```python
from build123d import *

# Parameters (mm, degrees)
SKETCH1_R             = 90
BOSS_EXTRUDE1_DEPTH   = 30
CUT_EXTRUDE4_DEPTH    = 30
SKETCH5_R             = 55.626023842
CUT_EXTRUDE5_DEPTH    = 30
SKETCH6_W             = 7.386739777
SKETCH6_H             = 13.542356258
CUT_EXTRUDE6_DEPTH    = 30
FILLET1_R             = 10
SKETCH8_R             = 10.49811893
BOSS_EXTRUDE2_DEPTH   = 30
BOSS_EXTRUDE2_2_DEPTH = 30
BOSS_EXTRUDE2_3_DEPTH = 30
BOSS_EXTRUDE2_4_DEPTH = 30
BOSS_EXTRUDE2_5_DEPTH = 30
BOSS_EXTRUDE4_DEPTH   = 30


with BuildPart() as part:
    # Sketch1 → Boss-Extrude1 (new body)
    with BuildSketch(Plane.XY):
        Circle(SKETCH1_R)
    extrude(amount=BOSS_EXTRUDE1_DEPTH)

    # Sketch4 → Cut-Extrude4 (cut)
    with BuildSketch(Plane.XY):
        with BuildLine():
            Line((88.736574157, 15.027322012), (45.122701232, 44.870398789))
            Line((45.122701232, 44.870398789), (52.120312028, 73.372154623))
            ThreePointArc((52.120312028, 73.372154623), (76.231197482, 47.84145201), (88.736574157, 15.027322012))
        make_face()
        with BuildLine():
            Line((41.712941959, -79.749799204), (56.61796667, -29.048523269))
            Line((56.61796667, -29.048523269), (85.887127938, -26.896119693))
            ThreePointArc((85.887127938, -26.896119693), (69.056660207, -57.716355404), (41.712941959, -79.749799204))
        make_face()
        with BuildLine():
            Line((-62.956558256, -64.315408516), (-10.130873456, -62.823373493))
            Line((-10.130873456, -62.823373493), (0.960852233, -89.994870759))
            ThreePointArc((0.960852233, -89.994870759), (-33.551834325, -83.512121356), (-62.956558256, -64.315408516))
        make_face()
        with BuildLine():
            Line((-80.622234776, 40.000690741), (-62.879190802, -9.778456837))
            Line((-62.879190802, -9.778456837), (-85.2932886, -28.723769249))
            ThreePointArc((-85.2932886, -28.723769249), (-89.792834204, 6.103025933), (-80.622234776, 40.000690741))
        make_face()
        with BuildLine():
            Line((13.129276916, 89.037194967), (-28.730603645, 56.77995481))
            Line((-28.730603645, 56.77995481), (-53.6750036, 72.242605078))
            ThreePointArc((-53.6750036, 72.242605078), (-21.943189159, 87.283998817), (13.129276916, 89.037194967))
        make_face()
    extrude(amount=CUT_EXTRUDE4_DEPTH, mode=Mode.SUBTRACT)

    # Sketch5 → Cut-Extrude5 (cut)
    with BuildSketch(Plane.XY):
        Circle(SKETCH5_R)
    extrude(amount=CUT_EXTRUDE5_DEPTH, mode=Mode.SUBTRACT)

    # Sketch6 → Cut-Extrude6 (cut)
    with BuildSketch(Plane.XY):
        with Locations((56.030331415, 2.229633356)):
            Rectangle(SKETCH6_W, SKETCH6_H)
    extrude(amount=CUT_EXTRUDE6_DEPTH, mode=Mode.SUBTRACT)

    # Fillet1
    fillet1_edges = [part.edges().sort_by_distance(p)[0] for p in [
        (85.887127938, -26.896119693, 15),
        (0.960852233, -89.994870759, 15),
        (-85.2932886, -28.723769249, 15),
        (-53.6750036, 72.242605078, 15),
        (52.120312028, 73.372154623, 15),
    ]]
    fillet(fillet1_edges, radius=FILLET1_R)



with BuildPart() as body_2:
    # Sketch8 → Boss-Extrude2 (new body)
    with BuildSketch(Plane.XY.offset(30)):
        with Locations((67.093562258, 42.627771692)):
            Circle(SKETCH8_R)
    extrude(amount=-BOSS_EXTRUDE2_DEPTH)


with BuildPart() as body_3:
    # Sketch8 → Boss-Extrude2 2 (new body)
    with BuildSketch(Plane.XY.offset(30)):
        with Locations((61.274470993, -50.637063702)):
            Circle(SKETCH8_R)
    extrude(amount=-BOSS_EXTRUDE2_2_DEPTH)


with BuildPart() as body_4:
    # Sketch8 → Boss-Extrude2 3 (new body)
    with BuildSketch(Plane.XY.offset(30)):
        with Locations((-29.223856541, -73.92319815)):
            Circle(SKETCH8_R)
    extrude(amount=-BOSS_EXTRUDE2_3_DEPTH)


with BuildPart() as body_5:
    # Sketch8 → Boss-Extrude2 4 (new body)
    with BuildSketch(Plane.XY.offset(30)):
        with Locations((-79.335807618, 4.950014688)):
            Circle(SKETCH8_R)
    extrude(amount=-BOSS_EXTRUDE2_4_DEPTH)


with BuildPart() as body_6:
    # Sketch8 → Boss-Extrude2 5 (new body)
    with BuildSketch(Plane.XY.offset(30)):
        with Locations((-19.808369092, 76.982475472)):
            Circle(SKETCH8_R)
    extrude(amount=-BOSS_EXTRUDE2_5_DEPTH)


with BuildPart() as part_1:
    add(part.part)

    add(body_2.part)  # Boss-Extrude4 merges body 2

    add(body_3.part)  # Boss-Extrude4 merges body 3

    add(body_4.part)  # Boss-Extrude4 merges body 4

    add(body_5.part)  # Boss-Extrude4 merges body 5

    add(body_6.part)  # Boss-Extrude4 merges body 6
    # Sketch9 → Boss-Extrude4 (add)
    with BuildSketch(Plane.XY):
        with BuildLine():
            Line((-29.298411126, 72.493644527), (-38.186452488, 62.641490221))
            Line((-38.186452488, 62.641490221), (-33.742460025, 59.886727574))
            Line((-33.742460025, 59.886727574), (-26.440954647, 68.84495067))
            ThreePointArc((-26.440954647, 68.84495067), (-28.073538286, 70.509649254), (-29.298411126, 72.493644527))
        make_face()
        with BuildLine():
            Line((46.528668919, 50.597003041), (57.304734615, 46.421101948))
            ThreePointArc((57.304734615, 46.421101948), (58.383460962, 48.48820141), (59.891846071, 50.266212961))
            Line((59.891846071, 50.266212961), (47.775334692, 55.674759504))
            Line((47.775334692, 55.674759504), (46.528668919, 50.597003041))
        make_face()
        with BuildLine():
            Line((62.498758869, -28.616059966), (61.857228356, -40.15513187))
            ThreePointArc((61.857228356, -40.15513187), (64.156501542, -40.54229273), (66.313607647, -41.427416431))
            Line((66.313607647, -41.427416431), (67.713233152, -28.232596532))
            Line((67.713233152, -28.232596532), (62.498758869, -28.616059966))
        make_face()
        with BuildLine():
            Line((-7.902311684, -68.282700724), (-19.074865041, -71.238338267))
            ThreePointArc((-19.074865041, -71.238338267), (-18.73256241, -73.544716298), (-18.907782629, -75.869764382))
            Line((-18.907782629, -75.869764382), (-5.926255116, -73.123463752))
            Line((-5.926255116, -73.123463752), (-7.902311684, -68.282700724))
        make_face()
        with BuildLine():
            Line((-67.382656079, -13.584969925), (-73.646143282, -3.872582481))
            ThreePointArc((-73.646143282, -3.872582481), (-75.733861807, -4.910841636), (-77.999259963, -5.462676675))
            Line((-77.999259963, -5.462676675), (-71.375860239, -16.960189442))
            Line((-71.375860239, -16.960189442), (-67.382656079, -13.584969925))
        make_face()
    extrude(amount=BOSS_EXTRUDE4_DEPTH)


solid = part_1.part
```
Geometry: final body of the model. Coordinates: model frame, mm. A direction names the side the tool comes from. Coordinates: 2 decimals unless noted, no trailing zeros. Order: outer loops, then holes, each group sorted by start corner. A loop starts at its lowest first (then second) coordinate and runs counter-clockwise, first axis right, second up. Notation, with made-up numbers: (26, -21.5) -> (56, -21.5) arc R20 cw to (56, 5.5) -> close; hole circle Ø2 at (44.5, 65). An arc over 180 degrees is marked (long way). Answer in a Markdown table with one row per item.
Item 1: Contact query for flat-ended pins moving along their axis: P1, Ø3, axis at x = -37.5, z = 11, coming from the -Y side; P2, Ø12, axis at y = 61.5, z = 12.5, coming from the +X side; P3, Ø6, axis at y = 9, z = 8.5, coming from the -X side; P4, Ø1, axis at x = -9, y = 54, coming from the -Z side. Output: stop coordinate, or through.
Return value:
| item | result |
|---|---|
| P1 | stops at y = -81.94 |
| P2 | stops at x = 50.62 |
| P3 | stops at x = -89.78 |
| P4 | passes through |
Item 2: Access query for faces 3 (the flat face through (57, 9.001, 15)), 4 (the flat face through (-12.508, -74.516, 14.79)), 5 (the flat face through (73.18, -27.83, 14.79)). Directions: +Z, -Z, +X, -X, +Y, -Y. A direction counts if a zero-diameter tool reaches every point of the face in a straight line with its end or side. Return the directions, or none.
Return value:
| item | result |
|---|---|
| face 3 | +Z, -Z |
| face 4 | +Z, -Z, -Y |
| face 5 | +Z, -Z, +X |
Item 3: Section B-B on y = 29.5. Output: boundary loops of the cut face in (x, z).
Return value:
| item | result |
|---|---|
| outline | (-76.88, 0) -> (-47.16, 0) -> (-47.16, 30) -> (-76.88, 30) -> close; (47.16, 0) -> (67.59, 0) -> (67.59, 30) -> (47.16, 30) -> close |
Item 4: Section D-D on x = -15. Output: boundary loops of the cut face in (y, z).
Return value:
| item | result |
|---|---|
| outline | (-75.04, 0) -> (-70.16, 0) -> (-70.16, 30) -> (-75.04, 30) -> close; (-62.96, 0) -> (-53.57, 0) -> (-53.57, 30) -> (-62.96, 30) -> close; (53.57, 0) -> (67.36, 0) -> (67.36, 30) -> (53.57, 30) -> close; (67.65, 0) -> (86.31, 0) -> (86.31, 30) -> (67.65, 30) -> close |
Item 5: Draft query along X for faces 1 (the cylindrical face through (25.34, -86.36, 14.79)), 2 (the flat face through (-33.68, 67.637, 14.79)). Return one class per face: released by +X, released by -X, zero draft, split by the parting line, or undercut.
Return value:
| item | result |
|---|---|
| face 1 | released by +X |
| face 2 | undercut |
Item 6: Section C-C on y = 2. Output: boundary loops of the cut face in (x, z).
Return value:
| item | result |
|---|---|
| outline | (-89.41, 0) -> (-69.26, 0) -> (-69.26, 30) -> (-89.41, 30) -> close; (-67.08, 0) -> (-55.59, 0) -> (-55.59, 30) -> (-67.08, 30) -> close; (59.72, 0) -> (89.98, 0) -> (89.98, 30) -> (59.72, 30) -> close |
Item 7: Section A-A on x = 17. Output: boundary loops of the cut face in (y, z), plus the area to 3 significant figures.
Return value:
| item | result |
|---|---|
| outline | (-88.38, 0) -> (-52.96, 0) -> (-52.96, 30) -> (-88.38, 30) -> close; (52.96, 0) -> (88.38, 0) -> (88.38, 30) -> (52.96, 30) -> close |
| area | 2,120 mm² |
Item 8: Ray query, L1, parallel to X at y = 0, z = 23.5; L2, parallel to X at y = -9, z = 25.75; L3, parallel to Y at x = 59.5, z = 14.5. Return the intervals inside material, ascending.
Return value:
| item | result |
|---|---|
| L1 | x = -88.59 to -70.08, -66.36 to -55.63, 59.72 to 90 |
| L2 | x = -75.96 to -70.34, -63.16 to -54.89, 54.89 to 89.55 |
| L3 | y = -60.98 to -40.29, -28.84 to -4.54, 9 to 35.03, 35.38 to 50.44 |
